The listing builds one solid part. Answer for the finished solid, in the listing's coordinates (mm). Coordinates: 2 decimals unless noted, no trailing zeros. Write each loop counter-clockwise with the first axis right and the second up, starting at its lowest first coordinate (ties: lowest second). Pieces come first, ordered by that corner, then holes.
(1) The part is cut by section B-B on z = 91.5. Determine the outline of the cut face in (x, y), plus the area to 3 significant figures.
(2) Given P1, Ø23.5, axis at x = 1170, y = 40, coming from the +Z side; P2, Ø4, axis at x = -659, y = 60.5, coming from the +Z side; P3, Ø2.5, axis at x = -1200.5, y = 95, coming from the +Z side, each flat-ended and moving along its own axis, determine where each tip first touches the part or whether it passes through.
(3) The part is cut by section A-A on x = 446.5. Determine the outline of the cut face in (y, z).
(4) Straight lines are drawn through the part: line 1 (Y direction, x = -160, z = 2.5); line 2 (Z direction, x = 1084.5, y = 57); line 3 (Y direction, x = -910, z = 58). For each, find the intervals that lie inside material, in ascending order.
from build123d import *

# Parameters (mm, degrees)
SKETCH_1_W          = 2440
SKETCH_1_H          = 100
SKETCH_1_R          = 13
EXTRUDE_710_DEPTH   = 8
SKETCH_2_W          = 2440
SKETCH_2_H          = 8
EXTRUDE_1_DEPTH     = 100
CUT_EXTRUDE_1_DEPTH = 1229.846613699


with BuildPart() as part:
    # 草图1 → Extrude 710 (new body)
    with BuildSketch(Plane.XY):
        with Locations((0, 50)):
            Rectangle(SKETCH_1_W, SKETCH_1_H)
        with Locations((1090, 40)):
            Circle(SKETCH_1_R, mode=Mode.SUBTRACT)
        with Locations((1170, 40)):
            Circle(SKETCH_1_R, mode=Mode.SUBTRACT)
        with Locations(Location((-1170, 40, 0), (0, 0, 180))):
            Circle(SKETCH_1_R, mode=Mode.SUBTRACT)
        with Locations(Location((-1090, 40, 0), (0, 0, 180))):
            Circle(SKETCH_1_R, mode=Mode.SUBTRACT)
        with Locations((0, 40)):
            Circle(SKETCH_1_R, mode=Mode.SUBTRACT)
        with Locations((80, 40)):
            Circle(SKETCH_1_R, mode=Mode.SUBTRACT)
        with Locations((160, 40)):
            Circle(SKETCH_1_R, mode=Mode.SUBTRACT)
        with Locations(Location((-160, 40, 0), (0, 0, 180))):
            Circle(SKETCH_1_R, mode=Mode.SUBTRACT)
        with Locations(Location((-80, 40, 0), (0, 0, 180))):
            Circle(SKETCH_1_R, mode=Mode.SUBTRACT)
    extrude(amount=EXTRUDE_710_DEPTH)

    # 草图2 → 凸台-拉伸1 (add)
    with BuildSketch(Plane.XY.offset(8)):
        with Locations((0, 96)):
            Rectangle(SKETCH_2_W, SKETCH_2_H)
    extrude(amount=EXTRUDE_1_DEPTH)

    # 草图3 → 切除-拉伸1 (cut, through all)
    with BuildSketch(Plane(origin=(0, 100, 0), x_dir=(-1, 0, 0), z_dir=(0, 1, 0))):
        Polygon((-1085, 108), (-1178, 15), (-1220, 15), (-1220, 108), align=None)
        Polygon((1220, 15), (1178, 15), (1085, 108), (1220, 108), align=None)
    extrude(amount=-CUT_EXTRUDE_1_DEPTH, mode=Mode.SUBTRACT)


solid = part.part
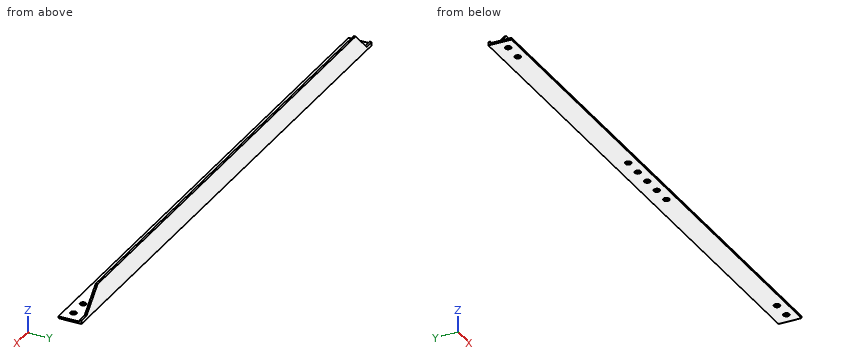
Model answer:
1. outline: (-1101.5, 92) - (1101.5, 92) - (1101.5, 100) - (-1101.5, 100) - close
1. area: 17,600 mm2
2. P1: passes through
2. P2: stops at z = 8
2. P3: stops at z = 15
3. outline: (0, 0) - (100, 0) - (100, 108) - (92, 108) - (92, 8) - (0, 8) - close
4. line 1: y = 0 to 27, 53 to 100
4. line 2: z = 0 to 8
4. line 3: y = 92 to 100
